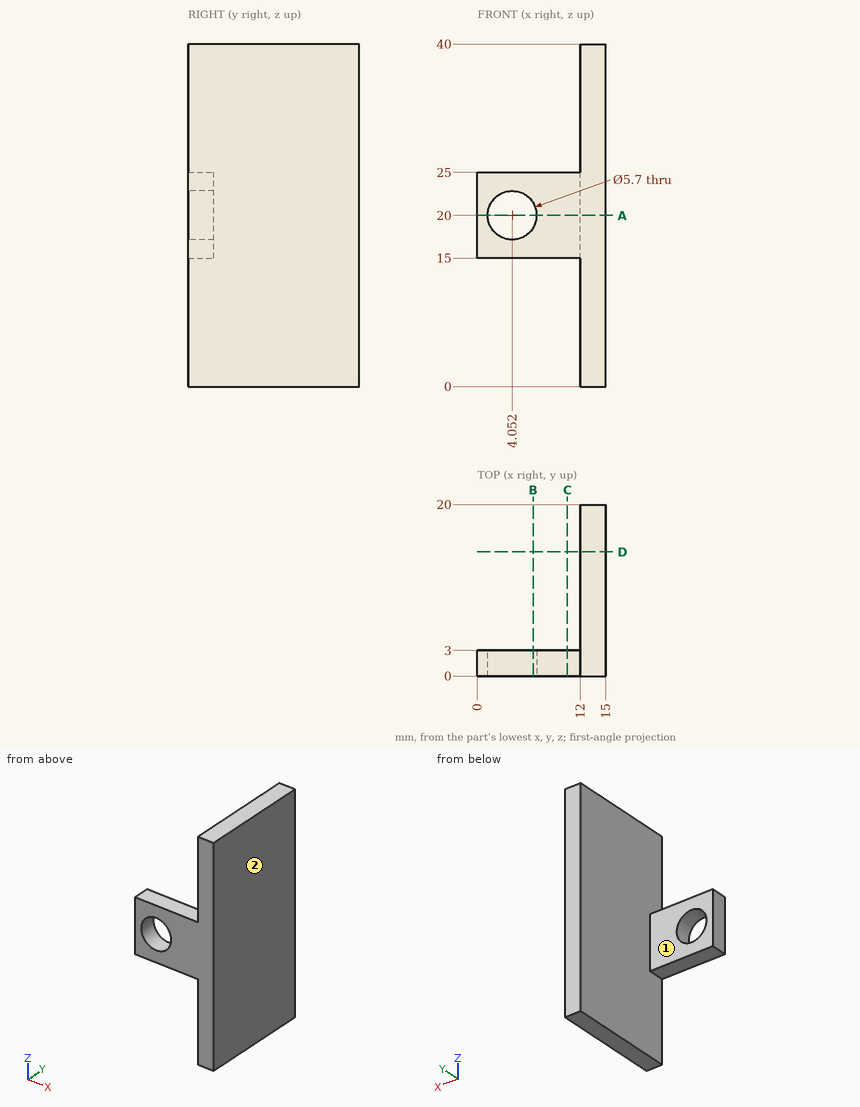
Here's the drawing with two shaded views (mm, measured from the low corner). I have some questions. A direction names the side the tool comes from. Coordinates: 2 decimals unless noted, no trailing zeros. Loops run counter-clockwise (first coordinate to the right, second up) from the corner with the lowest first, then second, coordinate; pieces in that order, holes last. Notation, with made-up numbers: (7, 39) -> (23, 39) arc R24 cw to (23, 70) -> close; hole circle Ø4 at (-36, 29). An arc over 180 degrees is marked (long way). Use one line per item in the form item = value. Start each with the question number.
(1) Will these pins go through, and if not, where does the flat tip stop? pin 1 (2 mm diameter, centred on y = 5, z = 19.5, fed in from -X); pin 2 (1.5 mm diameter, centred on x = 9, y = 1, fed in from +Z); pin 3 (4 mm diameter, centred on x = 2, z = 19.5, fed in from -Y); pin 4 (1.5 mm diameter, centred on x = 4, y = 1.5, fed in from -Z).
(2) If we section it at B-B (x = 6.5): Please give me the cut outline in (y, z).
(3) If we section it at D-D (y = 14.5): Please give me the cut outline in (x, z), then the cut area to 3 significant figures.
(4) On a 3-axis mill with a long thin cutter (end or side, diameter ignored), from which of +Z, -Z, +X, -X, +Y, -Y can I reach the whole of each face in a straight line? I mean the marked faces 1 and 2. Say none if no direction works.
(5) If we section it at A-A (z = 20): Please give me the cut outline in (x, y), then the cut area to 3 significant figures.
(6) Please list where this line runs through material, in increasing order: line 1 along X through (y, z) = (10.75, 38.5).
(7) If we section it at C-C (x = 10.5): Please give me the cut outline in (y, z), then the cut area to 3 significant figures.
Verdict:
q1.pin_1 = 12
q1.pin_2 = 25
q1.pin_3 = 0
q1.pin_4 = 15
q2.outline = (0, 15) -> (3, 15) -> (3, 18.54) -> (0, 18.54) -> close; (0, 21.46) -> (3, 21.46) -> (3, 25) -> (0, 25) -> close
q3.outline = (12, 0) -> (15, 0) -> (15, 40) -> (12, 40) -> close
q3.area = 120 mm²
q4.face_1 = +Z, -Z, -X, +Y
q4.face_2 = +Z, -Z, +X, +Y, -Y
q5.outline = (0, 0) -> (1.2, 0) -> (1.2, 3) -> (0, 3) -> close; (6.9, 0) -> (15, 0) -> (15, 20) -> (12, 20) -> (12, 3) -> (6.9, 3) -> close
q5.area = 78.9 mm²
q6.line_1 = 12 to 15
q7.outline = (0, 15) -> (3, 15) -> (3, 25) -> (0, 25) -> close
q7.area = 30.0 mm²
